from build123d import *

# Parameters (mm, degrees)
ESQUISSE1_W                       = 160
ESQUISSE1_H                       = 100
ESQUISSE1_W_2                     = 144
ESQUISSE1_H_2                     = 90
PROFONDEUR_BOITIER_DEPTH          = 46
ESQUISSE2_W                       = 144
ESQUISSE2_H                       = 90
PROFONDEUR_FOND_DEPTH             = 5
ESQUISSE3_W                       = 4
ESQUISSE3_H                       = 90
S_PARATION_PLATINE_BATTERIE_DEPTH = 42
ESQUISSE7_R                       = 3.3
ANTENNE_LORA_DEPTH                = 92
ESQUISSE8_W                       = 18.5
ESQUISSE8_H                       = 13
INTERRUPTEUR_DEPTH                = 92
ESQUISSE9_R                       = 3
VIS_PLATINE_DEPTH                 = 20
ESQUISSE10_W                      = 16.1
ESQUISSE10_H                      = 21
DHT22_DEPTH                       = 92
ESQUISSE11_W                      = 25
ESQUISSE11_H                      = 15
DB9_DEPTH                         = 92


with BuildPart() as part:
    # Esquisse1 → profondeur boitier (new body)
    with BuildSketch(Plane.XY):
        Rectangle(ESQUISSE1_W, ESQUISSE1_H)
        Rectangle(ESQUISSE1_W_2, ESQUISSE1_H_2, mode=Mode.SUBTRACT)
    extrude(amount=PROFONDEUR_BOITIER_DEPTH)

    # Esquisse2 → profondeur fond (add)
    with BuildSketch(Plane.XY):
        Rectangle(ESQUISSE2_W, ESQUISSE2_H)
    extrude(amount=PROFONDEUR_FOND_DEPTH)

    # Esquisse3 → Séparation platine batterie (add)
    with BuildSketch(Plane.XY):
        with Locations((40, 0)):
            Rectangle(ESQUISSE3_W, ESQUISSE3_H)
    extrude(amount=S_PARATION_PLATINE_BATTERIE_DEPTH)

    # Esquisse7 → Antenne LoRA (cut)
    with BuildSketch(Plane(origin=(0, 0, 0), x_dir=(0, 0, -1), z_dir=(1, 0, 0))):
        with Locations((-36, -20)):
            Circle(ESQUISSE7_R)
    extrude(amount=-ANTENNE_LORA_DEPTH, mode=Mode.SUBTRACT)

    # Esquisse8 → interrupteur (cut)
    with BuildSketch(Plane(origin=(0, 0, 0), x_dir=(1, 0, 0), z_dir=(0, 1, 0))):
        with Locations((10.75, -35)):
            Rectangle(ESQUISSE8_W, ESQUISSE8_H)
    extrude(amount=INTERRUPTEUR_DEPTH, mode=Mode.SUBTRACT)

    # Esquisse9 → Vis platine (add)
    with BuildSketch(Plane.XY):
        with Locations((-58.5, -32.5)):
            Circle(ESQUISSE9_R)
        with Locations((24.5, -32.5)):
            Circle(ESQUISSE9_R)
        with Locations((24.5, 32.5)):
            Circle(ESQUISSE9_R)
        with Locations((-58.5, 32.5)):
            Circle(ESQUISSE9_R)
    extrude(amount=VIS_PLATINE_DEPTH)

    # Esquisse10 → DHT22 (cut)
    with BuildSketch(Plane(origin=(0, 0, 0), x_dir=(1, 0, 0), z_dir=(0, 1, 0))):
        with Locations((-21.55, -33.5)):
            Rectangle(ESQUISSE10_W, ESQUISSE10_H)
    extrude(amount=DHT22_DEPTH, mode=Mode.SUBTRACT)

    # Esquisse11 → DB9 (cut)
    with BuildSketch(Plane(origin=(0, 0, 0), x_dir=(1, 0, 0), z_dir=(0, 1, 0))):
        with Locations((9.5, -32.5)):
            Rectangle(ESQUISSE11_W, ESQUISSE11_H)
    extrude(amount=-DB9_DEPTH, mode=Mode.SUBTRACT)


solid = part.part
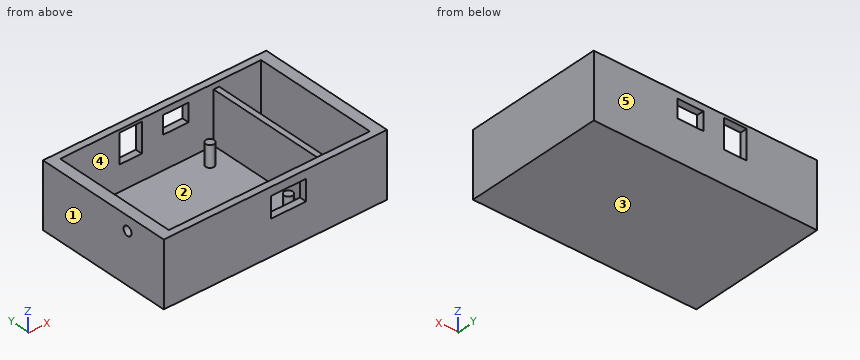
Geometry: final body of the model. Coordinates: model frame, mm. Face numbers are marked on the shaded views. A direction names the side the tool comes from. Coordinates: 2 decimals unless noted, no trailing zeros. Loops run counter-clockwise (first coordinate to the right, second up) from the corner with the lowest first, then second, coordinate; pieces in that order, holes last. Notation, with made-up numbers: (76.25, -9) - (121.25, -9) arc R8 cw to (121.25, 6) - close; hole circle Ø10 at (-9.5, 22). An arc over 180 degrees is marked (long way). One line per question, with ' | ' between items. Start each with the question number.
(1) Reachability of the marked faces 1 and 2 from +Z, -Z, +X, -X, +Y, -Y: full face, straight path, thin tool, end or side. Return the list, or none.
(2) Cut plane C-C on x = 10.5. Output: boundary loops of the cut face in (y, z).
(3) First-contact query: pin 1 (1.2 mm diameter, centred on x = 40.5, y = 22, fed in from +Z); pin 2 (3 mm diameter, centred on x = -59, y = 32.5, fed in from +Z). Flat tips, straight axial feed; report the tip coordinate or a pass-through.
(4) Ray query, L1, parallel to X at y = 13.5, z = 32; L2, parallel to Y at x = 71, z = 30; L3, parallel to Y at x = -74, z = 36. Return the intervals inside material, ascending. Write a range as from..to.
(5) Cut plane A-A on z = 36. Output: boundary loops of the cut face in (x, y).
(6) Cut plane B-B on y = -20. Output: boundary loops of the cut face in (x, z).
(7) Cut plane D-D on z = 7.5. Output: boundary loops of the cut face in (x, y), and give its area (3 significant figures).
(8) Draft query along Y for the marked faces 3, 4 and 5. Return one class per face: +Y half, -Y half, draft (parallel to the pull), parting line (faces both ways), or undercut.
Here are the results:
1) face 1: +Z, -Z, -X, +Y, -Y | face 2: +Z
2) outline: (-50, 0) - (50, 0) - (50, 28.5) - (45, 28.5) - (45, 5) - (-45, 5) - (-45, 25) - (-50, 25) - close; (-50, 40) - (-45, 40) - (-45, 46) - (-50, 46) - close; (45, 41.5) - (50, 41.5) - (50, 46) - (45, 46) - close
3) pin 1: z = 42 | pin 2: z = 20
4) L1: -80..-72, 38..42, 72..80 | L2: -50..-45, 45..50 | L3: -50..-23.3, -16.7..50
5) outline: (-80, -50) - (-3, -50) - (-3, -45) - (-72, -45) - (-72, -23.3) - (-80, -23.3) - close; (-80, -16.7) - (-72, -16.7) - (-72, 45) - (-29.6, 45) - (-29.6, 50) - (-80, 50) - close; (-13.5, 45) - (1.5, 45) - (1.5, 50) - (-13.5, 50) - close; (20, 45) - (38, 45) - (38, -45) - (22, -45) - (22, -50) - (80, -50) - (80, 50) - (20, 50) - close; hole (42, -45) - (72, -45) - (72, 45) - (42, 45) - close
6) outline: (-80, 0) - (80, 0) - (80, 46) - (72, 46) - (72, 5) - (42, 5) - (42, 42) - (38, 42) - (38, 5) - (-72, 5) - (-72, 32.7) - (-80, 32.7) - close; (-80, 39.3) - (-72, 39.3) - (-72, 46) - (-80, 46) - close
7) outline: (-80, -50) - (80, -50) - (80, 50) - (-80, 50) - close; circle Ø6 at (-58.5, -32.5); circle Ø6 at (-58.5, 32.5); circle Ø6 at (24.5, -32.5); circle Ø6 at (24.5, 32.5); hole (-72, -45) - (38, -45) - (38, 45) - (-72, 45) - close; hole (42, -45) - (72, -45) - (72, 45) - (42, 45) - close | area: 3,510 mm²
8) face 3: draft | face 4: undercut | face 5: +Y half
